Answer from the drawing. Dimensions are ordinates in mm from the lowest x, y and z of the part. A direction names the side the tool comes from. Give positions to 0.01 mm unless a question says otherwise; leave off trailing zeros. Write each loop counter-clockwise with the first axis right and the second up, starting at its lowest first coordinate (ties: lowest second). Pieces come first, ordered by that corner, then holes. Notation, with made-up numbers: M 64.25,74.25 L 103.25,74.25 A26 cw 103.25,102.25 Z; hole C 45.5,84.5 d3. An arc over 180 degrees is marked long. Answer as a JSON object with one key per item and string values.
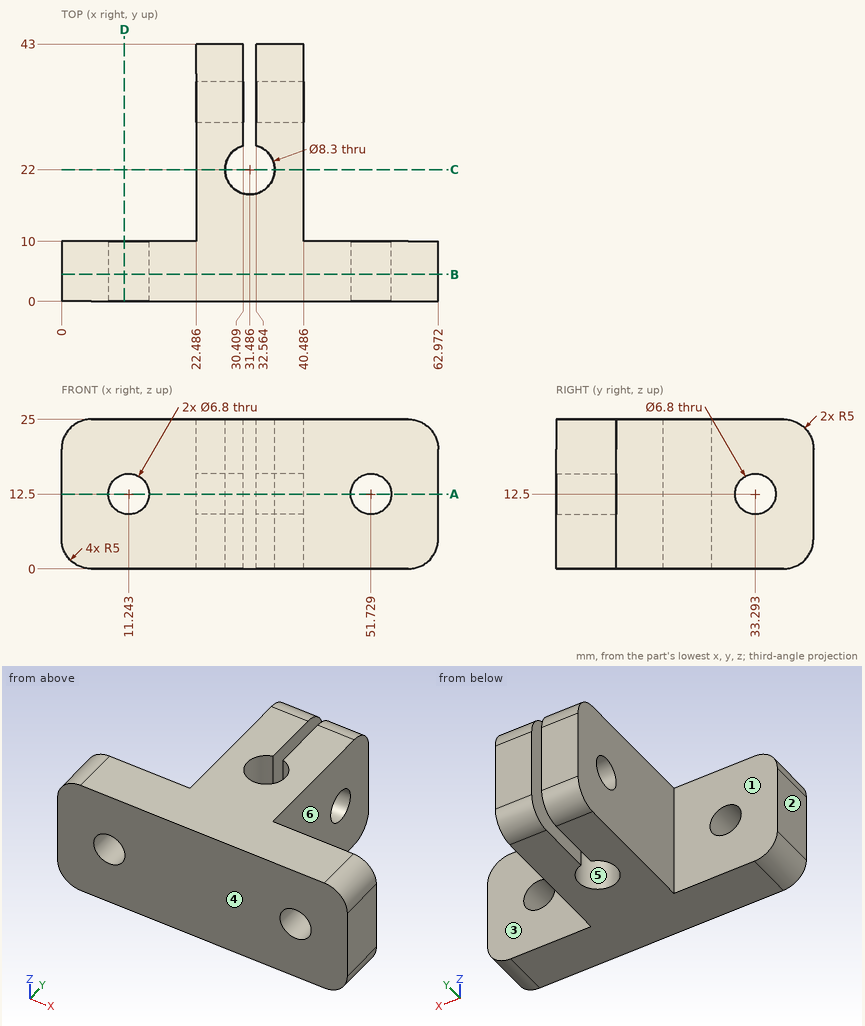
1. For the marked faces 1 and 2, determine the directions among +Z, -Z, +X, -X, +Y, -Y from which every point of the face is accessible in a straight line to the end or side of a thin tool.
Verdict:
{"face 1": "+Z, -Z, -X, +Y", "face 2": "+Z, -Z, -X, +Y, -Y"}
2. Flat-ended cylindrical pins translate along their axes: pin 1 (8.5 mm diameter, centred on y = 34, z = 11, fed in from -X); pin 2 (6 mm diameter, centred on x = 55, z = 13.5, fed in from +Y). Find the tip coordinate at first contact, or state that the pin passes through.
Verdict:
{"pin 1": "stops at x = 22.49", "pin 2": "stops at y = 10"}
3. Consider line 1 along Z through (x, y) = (26, 33); line 2 along X through (y, z) = (8, 11.5); line 3 along X through (y, z) = (22, 8.5). Determine where each line is inside the solid, lowest interval first.
Verdict:
{"line 1": "z = 0 to 9.11, 15.89 to 25", "line 2": "x = 0 to 7.99, 14.49 to 48.48, 54.98 to 62.97", "line 3": "x = 22.49 to 27.34, 35.64 to 40.49"}
4. A cutting plane is placed at C-C, the plane y = 22. Give the vertices of the cut face in (x, z).
Verdict:
{"outline": "M 22.49,0 L 27.34,0 L 27.34,25 L 22.49,25 Z; M 35.64,0 L 40.49,0 L 40.49,25 L 35.64,25 Z"}
5. The mould has two halves that part along Y. Classify the marked faces 3, 4, 5 and 6: released by +Y, released by -Y, zero draft, split by the parting line, or undercut.
Verdict:
{"face 3": "released by +Y", "face 4": "released by -Y", "face 5": "undercut", "face 6": "zero draft"}
6. A cutting plane is placed at B-B, the plane y = 4.5. Give the vertices of the cut face in (x, z).
Verdict:
{"outline": "M 0,5 A5 ccw 5,0 L 57.97,0 A5 ccw 62.97,5 L 62.97,20 A5 ccw 57.97,25 L 5,25 A5 ccw 0,20 Z; hole C 11.24,12.5 d6.8; hole C 51.73,12.5 d6.8"}
7. A cutting plane is placed at D-D, the plane x = 10.5. Give the vertices of the cut face in (y, z), plus the area to 3 significant figures.
Verdict:
{"outline": "M 0,0 L 10,0 L 10,9.18 L 0,9.18 Z; M 0,15.82 L 10,15.82 L 10,25 L 0,25 Z", "area": "184 mm2"}
8. A cutting plane is placed at A-A, the plane z = 12.5. Give the vertices of the cut face in (x, y).
Verdict:
{"outline": "M 0,0 L 7.84,0 L 7.84,10 L 0,10 Z; M 14.64,0 L 48.33,0 L 48.33,10 L 40.49,10 L 40.49,29.89 L 32.56,29.89 L 32.56,26.01 A4.15 cw long 30.41,26.01 L 30.41,29.89 L 22.49,29.89 L 22.49,10 L 14.64,10 Z; M 22.49,36.69 L 30.41,36.69 L 30.41,43 L 22.49,43 Z; M 32.56,36.69 L 40.49,36.69 L 40.49,43 L 32.56,43 Z; M 55.13,0 L 62.97,0 L 62.97,10 L 55.13,10 Z"}
